from build123d import *

# Parameters (mm, degrees)
SKETCH1_W                               = 130
SKETCH1_H                               = 100
BOSS_EXTRUDE1_DEPTH                     = 20
CUT_EXTRUDE1_DEPTH                      = 85.409715081
CUT_EXTRUDE1_DEPTH_BACK                 = 85.409715081
SKETCH11_R                              = 29
CBORE_FOR_M5_HEX_HEAD_BOLT2_D           = 5.5
CBORE_FOR_M5_HEX_HEAD_BOLT2_CBORE_D     = 10.5
CBORE_FOR_M5_HEX_HEAD_BOLT2_CBORE_DEPTH = 6
SKETCH15_R                              = 32.75
CUT_EXTRUDE2_DEPTH                      = 13
BOSS_EXTRUDE2_DEPTH                     = 65
BOSS_EXTRUDE2_DEPTH_BACK                = 65
SKETCH17_R                              = 42
CUT_EXTRUDE3_DEPTH                      = 85.409715081
CUT_EXTRUDE4_DEPTH                      = 85.409715081
CUT_EXTRUDE4_DEPTH_BACK                 = 2
SKETCH18_W                              = 10
SKETCH18_H                              = 3.5
SKETCH19_R                              = 3.25
CUT_EXTRUDE5_DEPTH                      = 90.162772501
CUT_EXTRUDE7_DEPTH                      = 11


with BuildPart() as part:
    # Sketch1 → Boss-Extrude1 (new body)
    with BuildSketch(Plane(origin=(0, 0, 0), x_dir=(1, 0, 0), z_dir=(0, 1, 0))):
        Rectangle(SKETCH1_W, SKETCH1_H)
    extrude(amount=BOSS_EXTRUDE1_DEPTH)

    # Sketch11 → Cut-Extrude1 (cut, two sides: drawn at the far end of the back side and taken through both)
    with BuildSketch(Plane(origin=(0, 20, 0), x_dir=(1, 0, 0), z_dir=(0, 1, 0)).offset(-CUT_EXTRUDE1_DEPTH_BACK)):
        with Locations(Location((0, 0, 0), (0, 0, 270))):
            Circle(SKETCH11_R)
    extrude(amount=CUT_EXTRUDE1_DEPTH + CUT_EXTRUDE1_DEPTH_BACK, mode=Mode.SUBTRACT)

    # CBORE for M5 Hex Head Bolt2 (through all)
    with Locations(Plane(origin=(-32.335783638, 20, -13.393920133), x_dir=(0, 0, 1), z_dir=(0, 1, 0))):
        with Locations((0, 0), (-18.941863505, 18.941863505), (-18.941863505, 45.729703771), (0, 64.671567276), (26.787840266, 64.671567276), (45.729703771, 45.729703771), (45.729703771, 18.941863505), (26.787840266, 0)):
            CounterBoreHole(CBORE_FOR_M5_HEX_HEAD_BOLT2_D / 2, CBORE_FOR_M5_HEX_HEAD_BOLT2_CBORE_D / 2, CBORE_FOR_M5_HEX_HEAD_BOLT2_CBORE_DEPTH)

    # Sketch15 → Cut-Extrude2 (cut)
    with BuildSketch(Plane(origin=(0, 0, 0), x_dir=(1, 0, 0), z_dir=(0, 1, 0))):
        Circle(SKETCH15_R)
    extrude(amount=CUT_EXTRUDE2_DEPTH, mode=Mode.SUBTRACT)

    # Sketch16 → Boss-Extrude2 (add, two sides: drawn at the far end of the back side and taken through both)
    with BuildSketch(Plane(origin=(0, 0, 0), x_dir=(0, 0, -1), z_dir=(1, 0, 0)).offset(-BOSS_EXTRUDE2_DEPTH_BACK)):
        Polygon((-50, 20), (-50, 35), (-30.3, 35), (-30.3, 30), (-35.3, 30), (-35.3, 20), align=None)
        Polygon((30.3, 35), (30.3, 30), (35.3, 30), (35.3, 20), (50, 20), (50, 35), align=None)
    extrude(amount=BOSS_EXTRUDE2_DEPTH + BOSS_EXTRUDE2_DEPTH_BACK)

    # Sketch17 → Cut-Extrude3 (cut, through all)
    with BuildSketch(Plane(origin=(0, 20, 0), x_dir=(1, 0, 0), z_dir=(0, 1, 0))):
        Circle(SKETCH17_R)
    extrude(amount=CUT_EXTRUDE3_DEPTH, mode=Mode.SUBTRACT)

    # Sketch18 → Cut-Extrude4 (cut, two sides: drawn at the far end of the back side and taken through both)
    with BuildSketch(Plane(origin=(0, 20, 0), x_dir=(1, 0, 0), z_dir=(0, 1, 0)).offset(-CUT_EXTRUDE4_DEPTH_BACK)):
        with Locations((-50, -37.05)):
            Rectangle(SKETCH18_W, SKETCH18_H)
        with Locations((50, -37.05)):
            Rectangle(SKETCH18_W, SKETCH18_H)
    extrude(amount=CUT_EXTRUDE4_DEPTH + CUT_EXTRUDE4_DEPTH_BACK, mode=Mode.SUBTRACT)

    # Sketch19 → Cut-Extrude5 (cut, through all)
    with BuildSketch(Plane.XY):
        with Locations((-50, 25)):
            Circle(SKETCH19_R)
        with Locations(Location((50, 25, 0), (0, 0, 180))):
            Circle(SKETCH19_R)
    extrude(amount=CUT_EXTRUDE5_DEPTH, mode=Mode.SUBTRACT)

    # Sketch21 → Cut-Extrude7 (cut)
    with BuildSketch(Plane.XZ):
        Polygon((0, 0), (-20.393190362, -56.02983003), (20.393190362, -56.02983003), align=None)
    extrude(amount=-CUT_EXTRUDE7_DEPTH, mode=Mode.SUBTRACT)


solid = part.part
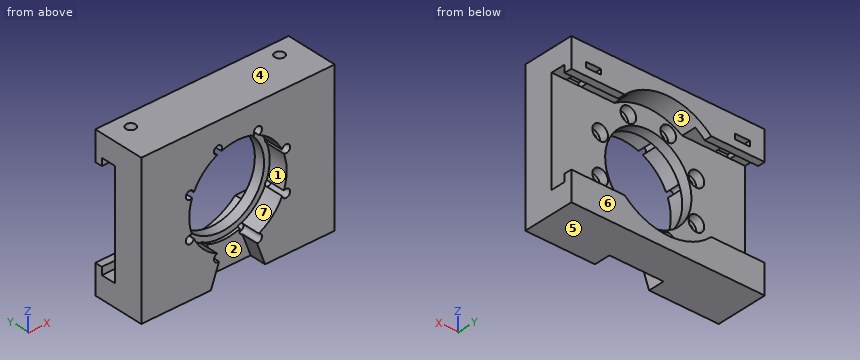
Part model, mm, in its own coordinate system. Face numbers are marked on the shaded views. A direction names the side the tool comes from. Give positions to 0.01 mm unless a question says otherwise; leave off trailing zeros. Order: outer loops, then holes, each group sorted by start corner. A loop starts at its lowest first (then second) coordinate and runs counter-clockwise, first axis right, second up. Notation, with made-up numbers: (59.5, -34) - (73.5, -34) arc R19 cw to (73.5, -29) - close; hole circle Ø7 at (-26.5, 4). An arc over 180 degrees is marked (long way). Use a Markdown table: item, result.
1) Saw through at A-A on y = 25. List the corners of the cut face in (x, z).
Checked values:
| item | result |
|---|---|
| outline | (-65, -50) - (65, -50) - (65, -35.3) - (22.76, -35.3) arc R42 cw to (-22.76, -35.3) - (-65, -35.3) - close; (-65, 35.3) - (-55, 35.3) - (-55, 38.8) - (-53.25, 38.8) - (-53.25, 50) - (-65, 50) - close; (-46.75, 38.8) - (-45, 38.8) - (-45, 35.3) - (-22.76, 35.3) arc R42 cw to (22.76, 35.3) - (45, 35.3) - (45, 38.8) - (46.75, 38.8) - (46.75, 50) - (-46.75, 50) - close; (53.25, 38.8) - (55, 38.8) - (55, 35.3) - (65, 35.3) - (65, 50) - (53.25, 50) - close |
2) Two-plate mould, pull along Z, no slides. Class the marked faces 5, 6 and 7: +Z half, -Z half, draft (parallel to the pull), parting line (faces both ways), or undercut.
Checked values:
| item | result |
|---|---|
| face 5 | -Z half |
| face 6 | draft |
| face 7 | undercut |
3) Probe L1, parallel to Z at x = -29.5, y = 22; L2, parallel to Z at x = -1, y = 24; L3, parallel to Y at x = 32, z = 33.5. List the from-to ranges inside material, lowest first. Write a range as from..to.
Checked values:
| item | result |
|---|---|
| L1 | -50..-35.3, 35.3..50 |
| L2 | -50..-41.99, 41.99..50 |
| L3 | 0..20, 30..35 |
4) Saw through at B-B on z = 0. List the corners of the cut face in (x, y).
Checked values:
| item | result |
|---|---|
| outline | (-65, 0) - (-32.75, 0) - (-32.75, 13) - (-29, 13) - (-29, 20) - (-65, 20) - close; (29, 13) - (32.75, 13) - (32.75, 0) - (65, 0) - (65, 20) - (29, 20) - close |
5) 3-axis set-ups, long thin cutter, end or side, ignore diameter. For the marked faces 1, 2, 3 and 4: which of +Z, -Z, +X, -X, +Y, -Y reach the whole face in a straight line?
Checked values:
| item | result |
|---|---|
| face 1 | -Y |
| face 2 | -Z, -Y |
| face 3 | +Y |
| face 4 | +Z, +X, -X, +Y, -Y |
6) Flat gauge pins, fed straight in: P1, Ø11.5, axis at x = -32.5, z = -12.5, coming from the +Y side; P2, Ø3, axis at x = 30.5, z = -14, coming from the +Y side; P3, Ø6.5, axis at x = -13.39, z = -32.34, coming from the -Y side; P4, Ø19.5, axis at x = 13.5, z = -15.5, coming from the -Y side. Where does each tip first touch, or does it go through?
Checked values:
| item | result |
|---|---|
| P1 | y = 20 |
| P2 | y = 14 |
| P3 | y = 0 |
| P4 | y = 13 |
7) Saw through at D-D on x = -6. List the corners of the cut face in (y, z), plus the area to 3 significant figures.
Checked values:
| item | result |
|---|---|
| outline | (0, 32.2) - (13, 32.2) - (13, 28.37) - (20, 28.37) - (20, 41.57) - (35, 41.57) - (35, 50) - (0, 50) - close; (11, -50) - (35, -50) - (35, -41.57) - (20, -41.57) - (20, -28.37) - (13, -28.37) - (13, -32.2) - (11, -32.2) - close |
| area | 823 mm² |
8) Saw through at C-C on x = -50. List the corners of the cut face in (y, z).
Checked values:
| item | result |
|---|---|
| outline | (0, -50) - (35, -50) - (35, -30.3) - (30, -30.3) - (30, -35.3) - (20, -35.3) - (20, 35.3) - (18, 35.3) - (18, 38.8) - (21.75, 38.8) - (21.75, 50) - (0, 50) - close; (28.25, 38.8) - (35, 38.8) - (35, 50) - (28.25, 50) - close; (30, 30.3) - (35, 30.3) - (35, 35.3) - (30, 35.3) - close |
